Geometry: see drawing. Coordinates: mm, zero at the bounding-box minimum. A direction names the side the tool comes from. Coordinates: 2 decimals unless noted, no trailing zeros. Loops run counter-clockwise (first coordinate to the right, second up) from the corner with the lowest first, then second, coordinate; pieces in that order, holes last. Notation, with made-up numbers: (27.5, 70) - (55.5, 70) arc R25 ccw to (55.5, 101) - close; hole circle Ø4 at (78.5, 39.25). An arc over 180 degrees is marked (long way). Use one line per item in the form item = value.
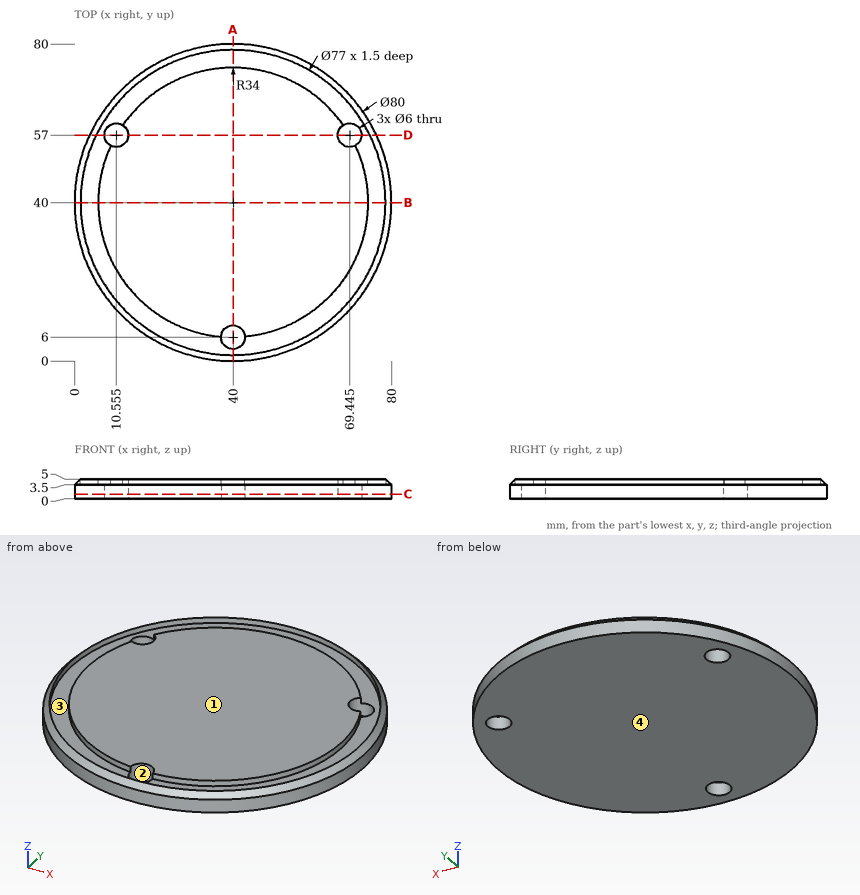
Q1. Cut plane A-A, the plane x = 40. Return loops of the section in (y, z), then the cut area to 3 significant figures.
Check values:
outline = (0, 0) - (3, 0) - (3, 3.5) - (1.5, 3.5) - (1.5, 5) - (0, 3.5) - close; (9, 0) - (80, 0) - (80, 3.5) - (78.5, 5) - (78.5, 3.5) - (74, 3.5) - (74, 5) - (9, 5) - close
area = 359 mm²
Q2. Cut plane B-B, the plane y = 40. Return loops of the section in (x, z).
Check values:
outline = (0, 0) - (80, 0) - (80, 3.5) - (78.5, 5) - (78.5, 3.5) - (74, 3.5) - (74, 5) - (6, 5) - (6, 3.5) - (1.5, 3.5) - (1.5, 5) - (0, 3.5) - close
Q3. Set-up query: the marked faces 3 and 4. Return all of +Z, -Z, +X, -X, +Y, -Y with unobstructed straight access to the full face (end or side cutting, diameter ignored); none if empty.
Check values:
face_3 = +Z
face_4 = -Z, +X, -X, +Y, -Y
Q4. Cut plane C-C, the plane z = 1.2. Return loops of the section in (x, y) (3 decimals).
Check values:
outline = circle Ø80 at (40, 40); hole circle Ø6 at (10.555, 57); hole circle Ø6 at (40, 6); hole circle Ø6 at (69.445, 57)
Q5. Pull-direction query (Y, two-part tool) for the marked faces 1 and 2; classes: pulls with the +Y half, pulls with the -Y half, needs draft (parallel to the pull), parting line crosses it, or undercut.
Check values:
face_1 = needs draft
face_2 = undercut
Q6. Cut plane D-D, the plane y = 57. Give the number of separate pieces and of enclosed holes in the cut face, then the cut area to 3 significant figures.
Check values:
separate_pieces = 3
enclosed_holes = 0
area = 293 mm²
Q7. Ray query, line 1 along Y through (x, z) = (60.5, 3.9) (1 decimal); line 2 along Y through (x, z) = (40, 1.55); line 3 along Y through (x, z) = (49, 4.55). Return the intervals inside material, ascending. Write a range as [from, to].
Check values:
line_1 = [6.1, 7.4], [12.9, 67.1], [72.6, 73.9]
line_2 = [0, 3], [9, 80]
line_3 = [2.1, 2.57], [7.21, 72.79], [77.43, 77.9]
Q8. First-contact query: P1, Ø3, axis at x = 49.5, z = 4, coming from the -Y side; P2, Ø8, axis at x = 69.44, y = 57, coming from the +Z side; P3, Ø2, axis at y = 68.5, z = 1.5, coming from the -X side; P4, Ø2, axis at x = 42.5, z = 1.5, coming from the -Y side. Flat tips, straight axial feed; report the tip coordinate or a pass-through.
Check values:
P1 = 0.83
P2 = 5
P3 = 10.95
P4 = 0.03
